Design review of the part shown in the three views and the two pictorial views. Dimensions are in mm from the part's minimum x, y and z. Round coordinates to 2 decimals unless told otherwise and drop trailing zeros. Loops run counter-clockwise (first coordinate to the right, second up) from the corner with the lowest first, then second, coordinate; pieces in that order, holes last. Notation, with made-up numbers: (-25, 79.25) -> (3, 79.25) arc R23 ccw to (3, 94.25) -> close; hole circle Ø10 at (73, 76). An arc over 180 degrees is marked (long way). One line per question, with ' | ' between items. Start each with the question number.
1. Consider section C-C (y = 5). Count the separate pieces of the cut face and the enclosed holes in it, and give its area (3 significant figures).
2. For pin 1 Ø1 at (x, y) = (17, 3) entering from -Z (1 decimal), flat-tipped, find the tip position at first contact; note if it passes through.
3. Consider section D-D (x = 25). Write out the cut boundary in (y, z).
4. Draft analysis for pull direction X (two halves, no side actions). For the marked faces 1, 2 and 3, state which applies: pulls with the +X half, pulls with the -X half, needs draft (parallel to the pull), parting line crosses it, or undercut.
5. Consider section A-A (z = 31). Write out the cut boundary in (x, y), and give its area (3 significant figures).
6. Wall thickness on line 1 along Z through (x, y) = (31, 3.5) (1 decimal); line 2 along Z through (x, y) = (33, 2) (1 decimal); line 3 along X through (y, z) = (3.25, 38.5): over which ranges is each line inside the solid? List them lowest first.
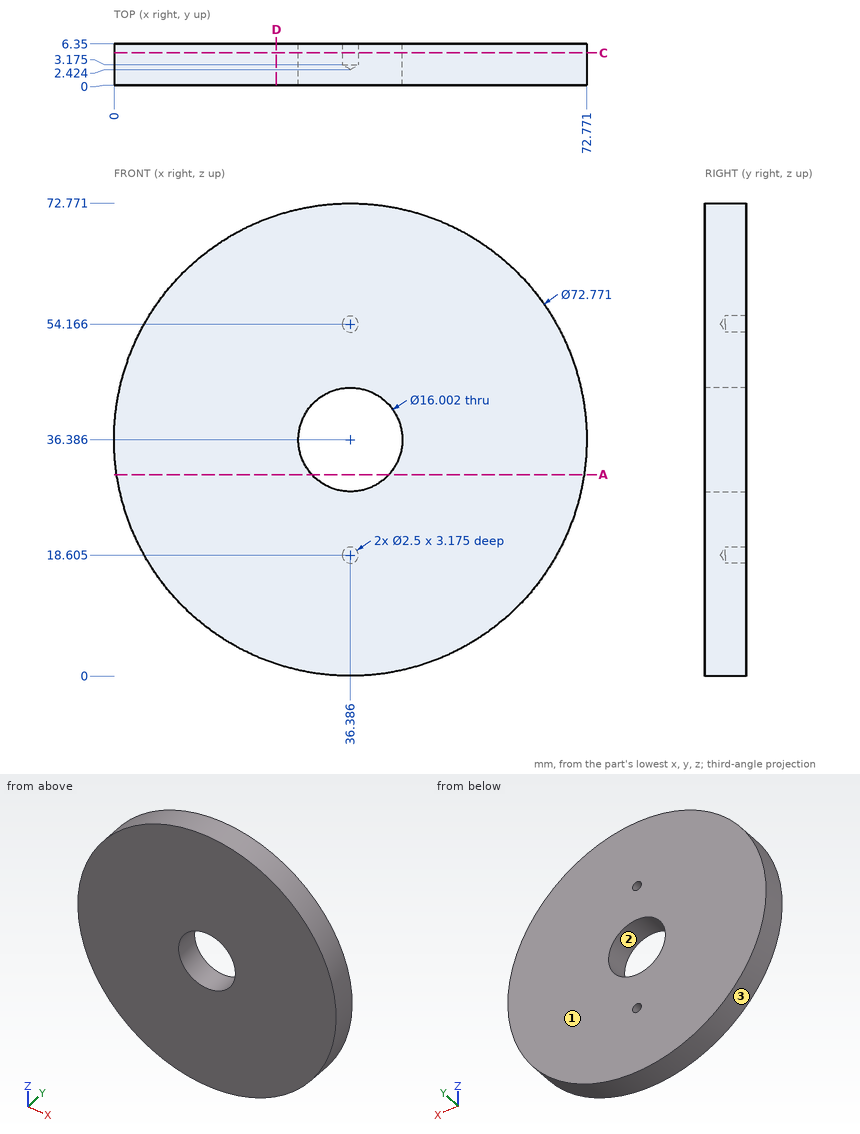
Answer block:
1) separate pieces: 1 | enclosed holes: 3 | area: 3,950 mm2
2) pin 1: stops at z = 5.3
3) outline: (0, 1.83) -> (6.35, 1.83) -> (6.35, 70.94) -> (0, 70.94) -> close
4) face 1: needs draft | face 2: undercut | face 3: parting line crosses it
5) outline: (0.4, 0) -> (30.47, 0) -> (30.47, 6.35) -> (0.4, 6.35) -> close; (42.3, 0) -> (72.37, 0) -> (72.37, 6.35) -> (42.3, 6.35) -> close | area: 382 mm2
6) line 1: z = 0.4 to 30.5, 42.3 to 72.4 | line 2: z = 0.2 to 29.1, 43.6 to 72.6 | line 3: x = 0.06 to 28.67, 44.1 to 72.71
